Here's how the part is built. I have some questions about the finished solid (model axes, mm). Face numbers are marked on the shaded views. A direction names the side the tool comes from. Give positions to 0.01 mm unless a question says otherwise; leave off trailing zeros. Loops run counter-clockwise (first coordinate to the right, second up) from the corner with the lowest first, then second, coordinate; pieces in that order, holes last. Notation, with made-up numbers: (33.25, 37) - (40.25, 37) arc R25 ccw to (40.25, 59) - close; hole circle Ø3 at (2, -1.5). An arc over 180 degrees is marked (long way). Put each result on its own line as item: value. Start each with the question number.
from build123d import *

# Parameters (mm, degrees)
SKETCH1_R           = 250
BOSS_EXTRUDE1_DEPTH = 125
SKETCH2_R           = 175
BOSS_EXTRUDE2_DEPTH = 100
SKETCH3_R           = 100
BOSS_EXTRUDE3_DEPTH = 400
SKETCH4_R           = 175
BOSS_EXTRUDE4_DEPTH = 150


with BuildPart() as part:
    # Sketch1 → Boss-Extrude1 (new body, symmetric)
    with BuildSketch(Plane(origin=(0, 0, 0), x_dir=(1, 0, 0), z_dir=(0, 1, 0))):
        Circle(SKETCH1_R)
    extrude(amount=BOSS_EXTRUDE1_DEPTH, both=True)

    # Sketch2 → Boss-Extrude2 (add)
    with BuildSketch(Plane.XZ.offset(125)):
        Circle(SKETCH2_R)
    extrude(amount=BOSS_EXTRUDE2_DEPTH)

    # Sketch3 → Boss-Extrude3 (add)
    with BuildSketch(Plane.XZ.offset(225)):
        Circle(SKETCH3_R)
    extrude(amount=BOSS_EXTRUDE3_DEPTH)

    # Sketch4 → Boss-Extrude4 (add)
    with BuildSketch(Plane.XZ.offset(625)):
        Circle(SKETCH4_R)
    extrude(amount=BOSS_EXTRUDE4_DEPTH)


solid = part.part
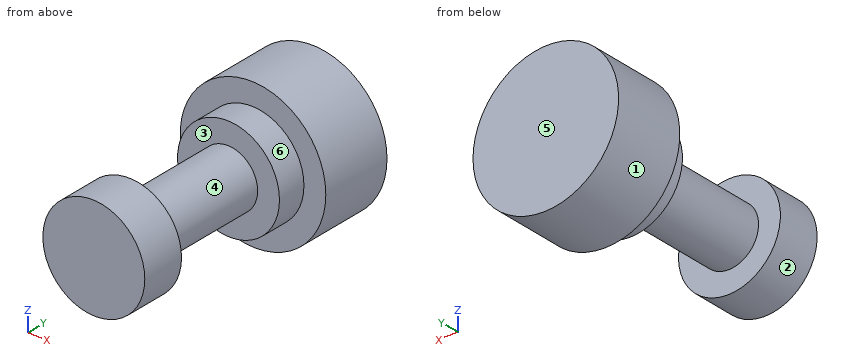
1) I need wall thicknesses on line 1 (Y direction, x = -10, z = -103.5); line 2 (Y direction, x = 171.5, z = 65); line 3 (Z direction, x = -1, y = -667). Which ranges of each line are inside material? Lowest first, please.
2) Suppose I cut it at C-C on x = -154.5. Please give me the cut outline in (y, z).
3) Thinking about a two-plate mould opening in Y: for the marked faces 4, 5 and 6, which applies, pulls with the +Y half, pulls with the -Y half, needs draft (parallel to the pull), parting line crosses it, or undercut?
4) I'm going to push flat-ended pins straight in: P1, Ø2, axis at x = 22, y = -54, coming from the -Z side; P2, Ø12, axis at y = -318, z = -96, coming from the +X side; P3, Ø1, axis at x = 190, y = -101.5, coming from the +Z side. Where does each tip first touch, or does it pass through?
5) Which directions (+Z, -Z, +X, -X, +Y, -Y) give clear straight access to the entire face, cutting with the end or side of a thin tool? Please do the marked faces 1, 2 and 3.
6) Suppose I cut it at D-D on y = -389. Please give me the cut outline in (x, z), plus the area to 3 significant figures.
7) Suppose I cut it at A-A on x = 0. Please give me the cut outline in (y, z).
8) Suppose I cut it at B-B on z = 0. Please give me the cut outline in (x, y).
Ans:
1. line 1: y = -775 to -625, -225 to 125
1. line 2: y = -125 to 125
1. line 3: z = -175 to 175
2. outline: (-775, -82.19) - (-625, -82.19) - (-625, 82.19) - (-775, 82.19) - close; (-225, -82.19) - (-125, -82.19) - (-125, -196.54) - (125, -196.54) - (125, 196.54) - (-125, 196.54) - (-125, 82.19) - (-225, 82.19) - close
3. face 4: undercut
3. face 5: pulls with the +Y half
3. face 6: needs draft
4. P1: stops at z = -249.12
4. P2: stops at x = 43.59
4. P3: stops at z = 163.06
5. face 1: +Y, -Y
5. face 2: -Y
5. face 3: none
6. outline: circle Ø200 at (0, 0)
6. area: 31,400 mm²
7. outline: (-775, -175) - (-625, -175) - (-625, -100) - (-225, -100) - (-225, -175) - (-125, -175) - (-125, -250) - (125, -250) - (125, 250) - (-125, 250) - (-125, 175) - (-225, 175) - (-225, 100) - (-625, 100) - (-625, 175) - (-775, 175) - close
8. outline: (-250, -125) - (-175, -125) - (-175, -225) - (-100, -225) - (-100, -625) - (-175, -625) - (-175, -775) - (175, -775) - (175, -625) - (100, -625) - (100, -225) - (175, -225) - (175, -125) - (250, -125) - (250, 125) - (-250, 125) - close
